```python
from build123d import *

# Parameters (mm, degrees)
F0_W      = 200
F0_H      = 100
F1_DEPTH  = 40
F2_W      = 210
F2_H      = 105
F2_W_2    = 200
F2_H_2    = 100
F3_DEPTH  = 5
F4_W      = 210
F4_H      = 105
F5_DEPTH  = 5
F6_W      = 210
F6_H      = 50
F7_DEPTH  = 5
F8_R      = 20
F9_DEPTH  = 5
F10_R     = 10
F11_DEPTH = 5
F12_R     = 5
F13_DEPTH = 5
F14_DEPTH = 5
F15_DEPTH = 5
F16_DEPTH = 5
F12_W     = 80
F12_H     = 20
F17_DEPTH = 3
F18_R     = 4.99999


# Not quite as in the source:
# - a fillet or chamfer is up to 0.001 mm smaller than in the source, because OpenCascade refuses the exact size


with BuildPart() as f1:
    # F0 (on Top) → F1 (new body)
    with BuildSketch(Plane.XY):
        with Locations((8.9475423098, -1.9630908966)):
            Rectangle(F0_W, F0_H)
    extrude(amount=F1_DEPTH)

    # F2 (on face) → F3 (join)
    with BuildSketch(Plane.XY.offset(40)):
        Polygon((113.9475423098, -56.9630908966), (113.9475423098, 48.0369091034), (108.9475423098, 48.0369091034), (108.9475423098, -51.9630908966), (-91.0524576902, -51.9630908966), (-91.0524576902, 48.0369091034), (-96.0524576902, 48.0369091034), (-96.0524576902, -56.9630908966), align=None)
        with Locations((8.9475423098, -4.4630908966)):
            Rectangle(F2_W, F2_H)
        with Locations((8.9475423098, -1.9630908966)):
            Rectangle(F2_W_2, F2_H_2)
    extrude(amount=F3_DEPTH)

    # F4 (on face) → F5 (join)
    with BuildSketch(Plane(origin=(0, 0, 0), x_dir=(1, 0, 0), z_dir=(0, 0, -1))):
        with Locations((8.9475423098, 4.4630908966)):
            Rectangle(F4_W, F4_H)
    extrude(amount=F5_DEPTH)

    # F6 (on face) → F7 (join)
    with BuildSketch(Plane(origin=(0, 48.0369091034, 0), x_dir=(-1, 0, 0), z_dir=(0, 1, 0))):
        with Locations((-8.9475423098, 20)):
            Rectangle(F6_W, F6_H)
    extrude(amount=F7_DEPTH)

    # F8 (on face) → F9 (join)
    with BuildSketch(Plane.XY.offset(45)):
        with Locations((-46.0524576902, 0)):
            Circle(F8_R)
    extrude(amount=F9_DEPTH)

    # F10 (on face) → F11 (join)
    with BuildSketch(Plane.XY.offset(50)):
        with Locations((-46.0524576902, 0)):
            Circle(F10_R)
    extrude(amount=F11_DEPTH)

    # F12 (on face) → F13 (join)
    with BuildSketch(Plane.XZ.offset(51.9630908966)):
        with Locations((-78.6770284176, 20)):
            Circle(F12_R)
    extrude(amount=F13_DEPTH)

    # F12 (on face) → F14 (join)
    with BuildSketch(Plane.XZ.offset(51.9630908966)):
        with Locations((-58.6770284176, 20)):
            Circle(F12_R)
    extrude(amount=F14_DEPTH)

    # F12 (on face) → F15 (join)
    with BuildSketch(Plane.XZ.offset(51.9630908966)):
        with Locations((-38.6770284176, 19.7612177581)):
            Circle(F12_R)
    extrude(amount=F15_DEPTH)

    # F12 (on face) → F16 (join)
    with BuildSketch(Plane.XZ.offset(51.9630908966)):
        with Locations((-18.6770284176, 19.7612177581)):
            Circle(F12_R)
    extrude(amount=F16_DEPTH)

    # F12 (on face) → F17 (join)
    with BuildSketch(Plane.XZ.offset(51.9630908966)):
        with Locations((43.1329405028, 20)):
            Rectangle(F12_W, F12_H)
    extrude(amount=F17_DEPTH)

    # F18 (radius 5 in the source; OpenCascade refuses exactly that, so slightly less here)
    f18_edges = [f1.edges().sort_by_distance(p)[0] for p in [
        (8.947542, -56.963091, 45),
    ]]
    fillet(f18_edges, radius=F18_R)


solid = f1.part
```
Source: CAD feature listing. Evaluate the final solid. Frame: model axes, mm. A direction names the side the tool comes from. Round coordinates to 2 decimals unless told otherwise and drop trailing zeros. Loops run counter-clockwise (first coordinate to the right, second up) from the corner with the lowest first, then second, coordinate; pieces in that order, holes last. Notation, with made-up numbers: M 32,50.5 L 44,50.5 A10 ccw 44,62.5 Z; hole C 40,76.5 d10. An arc over 180 degrees is marked long. Use a Markdown table: item, result. Add a question column.
1. Reachability of faces 1 (the cylindrical face through (-66.033, 0.879, 47.465)), 2 (the flat face through (-94, 48.037, 20)), 3 (the flat face through (108.948, -3, 20)) from +Z, -Z, +X, -X, +Y, -Y: full face, straight path, thin tool, end or side. Return the list, or none.
2. Line query: line 1 (X direction, y = 29.5, z = 35.5); line 2 (Y direction, x = 58, z = 8); line 3 (Z direction, x = -6.5, y = -52). Output: solid intervals per line, ascending.
3. Mould query, pull axis X, two halves, no side actions, for faces 4 (the cylindrical face through (-62.645, -54.428, 16.958)), 5 (the flat face through (113.948, 5.9, -0.5)), 6 (the flat face through (-96.052, 5.9, -0.5)). Classes: pulls with the +X half, pulls with the -X half, needs draft (parallel to the pull), parting line crosses it, or undercut.
4. Contact query for flat-ended pins moving along their axis: P1, Ø10, axis at y = -36, z = 33.5, coming from the -X side; P2, Ø1.5, axis at y = -53.5, z = 17, coming from the +X side; P3, Ø16, axis at x = 44.5, z = 19.5, coming from the -Y side. Output: stop coordinate, or through.
5. Section query C-C on z = 34.5. Return the cut outline in (x, y).
6. Section query B-B on y = 0. Return the cut outline in (x, z).
Reported:
| question | item | result |
|---|---|---|
| 1 | face 1 | +Z |
| 1 | face 2 | -X, -Y |
| 1 | face 3 | +X, -Y |
| 2 | line 1 | x = -91.05 to 108.95 |
| 2 | line 2 | y = -51.96 to 53.04 |
| 2 | line 3 | z = -5 to 0, 40 to 45 |
| 3 | face 4 | undercut |
| 3 | face 5 | pulls with the +X half |
| 3 | face 6 | pulls with the -X half |
| 4 | P1 | stops at x = -91.05 |
| 4 | P2 | stops at x = 83.13 |
| 4 | P3 | stops at y = -54.96 |
| 5 | outline | M -96.05,48.04 L -91.05,48.04 L -91.05,-51.96 L 108.95,-51.96 L 108.95,48.04 L 113.95,48.04 L 113.95,53.04 L -96.05,53.04 Z |
| 6 | outline | M -96.05,-5 L 113.95,-5 L 113.95,0 L 108.95,0 L 108.95,40 L 113.95,40 L 113.95,45 L -26.05,45 L -26.05,50 L -36.05,50 L -36.05,55 L -56.05,55 L -56.05,50 L -66.05,50 L -66.05,45 L -96.05,45 L -96.05,40 L -91.05,40 L -91.05,0 L -96.05,0 Z |
